from build123d import *

# Parameters (mm, degrees)
CROQUIS1_W              = 74
CROQUIS1_H              = 80
SALIENTE_EXTRUIR1_DEPTH = 5
CROQUIS2_W              = 10
CROQUIS2_H              = 10
CROQUIS2_R              = 2.75
CROQUIS2_R_2            = 2.55
SALIENTE_EXTRUIR2_DEPTH = 10


with BuildPart() as part:
    # Croquis1 → Saliente-Extruir1 (new body)
    with BuildSketch(Plane.XY):
        with Locations((-29.301889279, 1.236374696)):
            Rectangle(CROQUIS1_W, CROQUIS1_H)
    extrude(amount=SALIENTE_EXTRUIR1_DEPTH)

    # Croquis2 → Saliente-Extruir2 (add)
    with BuildSketch(Plane.XY.offset(5)):
        with Locations((-61.301889279, 36.236374696)):
            Rectangle(CROQUIS2_W, CROQUIS2_H)
        with Locations((-61.301889279, 36.236374696)):
            Circle(CROQUIS2_R, mode=Mode.SUBTRACT)
        with Locations((2.698110721, 36.236374696)):
            Rectangle(CROQUIS2_W, CROQUIS2_H)
        with Locations((2.698110721, 36.236374696)):
            Circle(CROQUIS2_R, mode=Mode.SUBTRACT)
        with Locations((2.698110721, -33.763625304)):
            Rectangle(CROQUIS2_W, CROQUIS2_H)
        with Locations((2.698110721, -33.763625304)):
            Circle(CROQUIS2_R_2, mode=Mode.SUBTRACT)
        with Locations((-61.301889279, -33.763625304)):
            Rectangle(CROQUIS2_W, CROQUIS2_H)
        with Locations((-61.301889279, -33.763625304)):
            Circle(CROQUIS2_R_2, mode=Mode.SUBTRACT)
    extrude(amount=SALIENTE_EXTRUIR2_DEPTH)


solid = part.part
Geometry: final body of the model. Coordinates: model frame, mm. A direction names the side the tool comes from. Give positions to 0.01 mm unless a question says otherwise; leave off trailing zeros. Write each loop counter-clockwise with the first axis right and the second up, starting at its lowest first coordinate (ties: lowest second). Pieces come first, ordered by that corner, then holes. Notation, with made-up numbers: M -13,68.5 L 17,68.5 A21 ccw 17,94.5 Z; hole C -22,60.25 d5. An arc over 180 degrees is marked long. Answer in a Markdown table with one row per item. Add a question column.
(1) Reachability of faces 1 (the flat face through (-56.302, 36, 10)), 2 (the cylindrical face through (-59.824, 38.555, 9.93)), 3 (the flat face through (-61, 31.236, 10)) from +Z, -Z, +X, -X, +Y, -Y: full face, straight path, thin tool, end or side. Return the list, or none.
(2) Mould query, pull axis X, two halves, no side actions, for faces 4 (the flat face through (0, 39, 15)), 5 (the cylindrical face through (2.34, 38.963, 9.93)), 6 (the flat face through (7.698, 1, 4)). Classes: +X half, -X half, draft (parallel to the pull), parting line (faces both ways), or undercut.
(3) Section A-A on z = 7.5. Return loops of the section in (x, y), and give its area (3 significant figures).
(4) Section B-B on x = 3. Return loops of the section in (y, z), and give its area (3 significant figures).
(5) Section D-D on x = -7.5. Return loops of the section in (y, z), and give its area (3 significant figures).
(6) Ray query, line 1 (X direction, y = 33, z = 14.75); line 2 (Y direction, x = -2, z = 12.5); line 3 (Z direction, x = -14.5, y = -8). Return the intervals inside material, ascending.
(7) First-contact query: pin 1 (12 mm diameter, centred on x = -14, y = -8.5, fed in from +Z). Flat tip, straight axial feed; report the tip coordinate or a pass-through.
(8) Section C-C on y = -10.5. Return loops of the section in (x, z).
Result set:
| question | item | result |
|---|---|---|
| 1 | face 1 | +Z, +Y, -Y |
| 1 | face 2 | +Z |
| 1 | face 3 | +Z, +X, -X |
| 2 | face 4 | draft |
| 2 | face 5 | undercut |
| 2 | face 6 | +X half |
| 3 | outline | M -66.3,-38.76 L -56.3,-38.76 L -56.3,-28.76 L -66.3,-28.76 Z; M -66.3,31.24 L -56.3,31.24 L -56.3,41.24 L -66.3,41.24 Z; M -2.3,-38.76 L 7.7,-38.76 L 7.7,-28.76 L -2.3,-28.76 Z; M -2.3,31.24 L 7.7,31.24 L 7.7,41.24 L -2.3,41.24 Z; hole C -61.3,36.24 d5.5; hole C -61.3,-33.76 d5.1; hole C 2.7,36.24 d5.5; hole C 2.7,-33.76 d5.1 |
| 3 | area | 312 mm^2 |
| 4 | outline | M -38.76,0 L 41.24,0 L 41.24,15 L 38.97,15 L 38.97,5 L 33.5,5 L 33.5,15 L 31.24,15 L 31.24,5 L -28.76,5 L -28.76,15 L -31.23,15 L -31.23,5 L -36.3,5 L -36.3,15 L -38.76,15 Z |
| 4 | area | 495 mm^2 |
| 5 | outline | M -38.76,0 L 41.24,0 L 41.24,5 L -38.76,5 Z |
| 5 | area | 400 mm^2 |
| 6 | line 1 | x = -66.3 to -56.3, -2.3 to 7.7 |
| 6 | line 2 | y = -38.76 to -28.76, 31.24 to 41.24 |
| 6 | line 3 | z = 0 to 5 |
| 7 | pin 1 | stops at z = 5 |
| 8 | outline | M -66.3,0 L 7.7,0 L 7.7,5 L -66.3,5 Z |
